from build123d import *

# Parameters (mm, degrees)
ESQUISSE1_R        = 1.6
BOSS_EXTRU_1_DEPTH = 1.6
CHANFREIN1_SIZE    = 0.2
CHANFREIN1_SIZE2   = 0.549495484
CHANFREIN2_SIZE    = 0.2
CHANFREIN2_SIZE2   = 0.549495484
ESQUISSE4_W        = 6.573690578
ESQUISSE4_H        = 5.811523554
BOSS_EXTRU_2_DEPTH = 2.5
ESQUISSE5_W        = 2.839601435
ESQUISSE5_H        = 2.289720849
ESQUISSE5_W_2      = 2.157836197
ESQUISSE5_H_2      = 2.945915503
ESQUISSE5_W_3      = 2.645694815
ESQUISSE5_H_3      = 1.363110326
ESQUISSE5_W_4      = 3.433774122
ESQUISSE5_H_4      = 3.640175845
ESQUISSE5_W_5      = 2.683222401
ESQUISSE5_H_5      = 0.956953443
BOSS_EXTRU_3_DEPTH = 2


with BuildPart() as part:
    # Esquisse1 → Boss.-Extru.1 (new body)
    with BuildSketch(Plane(origin=(0, 0, 0), x_dir=(1, 0, 0), z_dir=(0, 1, 0))):
        with BuildLine():
            Line((16.1, -18.1), (-16.1, -18.1))
            ThreePointArc((-16.1, -18.1), (-17.514213562, -17.514213562), (-18.1, -16.1))
            Line((-18.1, -16.1), (-18.1, 16.1))
            ThreePointArc((-18.1, 16.1), (-17.514213562, 17.514213562), (-16.1, 18.1))
            Line((-16.1, 18.1), (16.1, 18.1))
            ThreePointArc((16.1, 18.1), (17.514213562, 17.514213562), (18.1, 16.1))
            Line((18.1, 16.1), (18.1, -16.1))
            ThreePointArc((18.1, -16.1), (17.514213562, -17.514213562), (16.1, -18.1))
        make_face()
        with Locations((-15.25, 15.25)):
            Circle(ESQUISSE1_R, mode=Mode.SUBTRACT)
        with Locations((15.25, 15.25)):
            Circle(ESQUISSE1_R, mode=Mode.SUBTRACT)
        with Locations((15.25, -15.25)):
            Circle(ESQUISSE1_R, mode=Mode.SUBTRACT)
        with Locations((-15.25, -15.25)):
            Circle(ESQUISSE1_R, mode=Mode.SUBTRACT)
    extrude(amount=BOSS_EXTRU_1_DEPTH)

    # Chanfrein1
    chanfrein1_edges = [part.edges().sort_by_distance(p)[0] for p in [
        (17.514213562, 1.6, -17.514213562),
        (0, 1.6, -18.1),
        (-17.514213562, 1.6, -17.514213562),
        (-18.1, 1.6, 0),
        (-17.514213562, 1.6, 17.514213562),
        (0, 1.6, 18.1),
        (17.514213562, 1.6, 17.514213562),
        (18.1, 1.6, 0),
    ]]
    chanfrein1_side = [part.faces().sort_by_distance(p)[0] for p in [
        (0, 1.6, 0),
    ]]
    chamfer(chanfrein1_edges, length=CHANFREIN1_SIZE, length2=CHANFREIN1_SIZE2, reference=chanfrein1_side[0])

    # Chanfrein2
    chanfrein2_edges = [part.edges().sort_by_distance(p)[0] for p in [
        (18.1, 0, 0),
        (17.514213562, 0, 17.514213562),
        (0, 0, 18.1),
        (-17.514213562, 0, 17.514213562),
        (-18.1, 0, 0),
        (-17.514213562, 0, -17.514213562),
        (0, 0, -18.1),
        (17.514213562, 0, -17.514213562),
    ]]
    chanfrein2_side = [part.faces().sort_by_distance(p)[0] for p in [
        (0, 0, 0),
    ]]
    chamfer(chanfrein2_edges, length=CHANFREIN2_SIZE, length2=CHANFREIN2_SIZE2, reference=chanfrein2_side[0])

    # Esquisse4 → Boss.-Extru.2 (add)
    with BuildSketch(Plane(origin=(0, 1.6, 0), x_dir=(1, 0, 0), z_dir=(0, 1, 0))):
        with Locations((-6.049700749, -4.854717359)):
            Rectangle(ESQUISSE4_W, ESQUISSE4_H)
    extrude(amount=BOSS_EXTRU_2_DEPTH)

    # Esquisse5 → Boss.-Extru.3 (add)
    with BuildSketch(Plane(origin=(0, 1.6, 0), x_dir=(1, 0, 0), z_dir=(0, 1, 0))):
        with Locations((1.628867377, 4.102355057)):
            Rectangle(ESQUISSE5_W, ESQUISSE5_H)
        with Locations((5.922641632, 3.492800834)):
            Rectangle(ESQUISSE5_W_2, ESQUISSE5_H_2)
        with Locations((1.531914066, 0.681555163)):
            Rectangle(ESQUISSE5_W_3, ESQUISSE5_H_3)
        with Locations((1.49438648, -3.384129307)):
            Rectangle(ESQUISSE5_W_4, ESQUISSE5_H_4)
        with Locations((-7.080666928, 4.487281863)):
            Rectangle(ESQUISSE5_W_5, ESQUISSE5_H_5)
    extrude(amount=BOSS_EXTRU_3_DEPTH)


solid = part.part
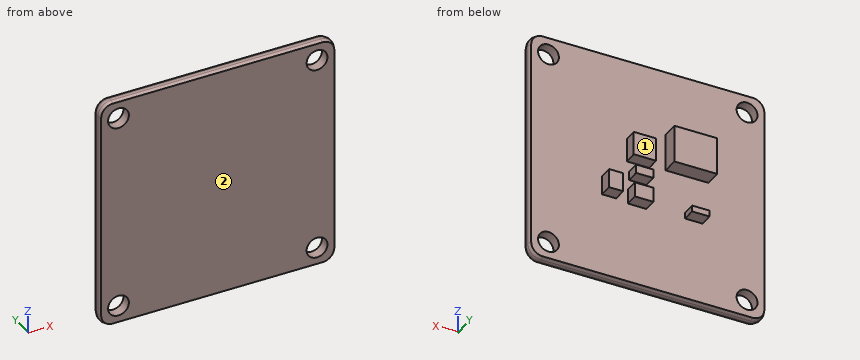
Build history of the part. All positions in model axes, mm. Face numbers are marked on the shaded views. A direction names the side the tool comes from. Round coordinates to 2 decimals unless told otherwise and drop trailing zeros. Loops run counter-clockwise (first coordinate to the right, second up) from the corner with the lowest first, then second, coordinate; pieces in that order, holes last. Notation, with made-up numbers: (72, -37) -> (92, -37) arc R15 ccw to (92, -12) -> close; hole circle Ø11 at (56, -27.75). An arc over 180 degrees is marked (long way). Answer in a Markdown table with one row per item.
Item 1: Which spindle directions (+Z, -Z, +X, -X, +Y, -Y) get a long thin tool onto all of the face, cutting with end or side? Do the marked faces 1 and 2. Say none if no direction does.
Answers below:
| item | result |
|---|---|
| face 1 | +Z, -Z, +X, +Y |
| face 2 | +Z, -Z, +X, -X, -Y |
Item 2: Drill centre lines: L1, parallel to X at y = 0.95, z = -15.25; L2, parallel to Z at x = 1.5, y = 3.2. Where is each one in solid material? Low to high. Write a range as [from, to].
Answers below:
| item | result |
|---|---|
| L1 | x = [-18.1, -16.85], [-13.65, 13.65], [16.85, 18.1] |
| L2 | z = [-5.25, -2.96], [-1.36, 0], [1.56, 5.2] |
Item 3: Saw through at C-C (z = 15.25). Write the cut outline in (x, y), and give its area (3 significant figures).
Answers below:
| item | result |
|---|---|
| outline | (-18.1, 0.55) -> (-17.9, 0) -> (-16.85, 0) -> (-16.85, 1.6) -> (-17.9, 1.6) -> (-18.1, 1.05) -> close; (-13.65, 0) -> (13.65, 0) -> (13.65, 1.6) -> (-13.65, 1.6) -> close; (16.85, 0) -> (17.9, 0) -> (18.1, 0.55) -> (18.1, 1.05) -> (17.9, 1.6) -> (16.85, 1.6) -> close |
| area | 47.5 mm² |
Item 4: Saw through at A-A (y = 3.1). Write the cut outline in (x, z).
Answers below:
| item | result |
|---|---|
| outline | (-9.34, 1.95) -> (-2.76, 1.95) -> (-2.76, 7.76) -> (-9.34, 7.76) -> close; (-8.42, -4.97) -> (-5.74, -4.97) -> (-5.74, -4.01) -> (-8.42, -4.01) -> close; (-0.22, 1.56) -> (3.21, 1.56) -> (3.21, 5.2) -> (-0.22, 5.2) -> close; (0.21, -5.25) -> (3.05, -5.25) -> (3.05, -2.96) -> (0.21, -2.96) -> close; (0.21, -1.36) -> (2.85, -1.36) -> (2.85, 0) -> (0.21, 0) -> close; (4.84, -4.97) -> (7, -4.97) -> (7, -2.02) -> (4.84, -2.02) -> close |
Item 5: Pin check, flat tips, straight feed: pin 1 (0.6 mm diameter, centred on y = 2, z = -4, fed in from -X); pin 2 (2 mm diameter, centred on y = 2.5, z = -8, fed in from -X); pin 3 (2 mm diameter, centred on x = -2, z = -2, fed in from -Y); pin 4 (1.6 mm diameter, centred on y = 2.5, z = 2.5, fed in from -X). Stop position of each tip, or through.
Answers below:
| item | result |
|---|---|
| pin 1 | stops at x = -8.42 |
| pin 2 | stops at x = -17.94 |
| pin 3 | stops at y = 0 |
| pin 4 | stops at x = -9.34 |
Item 6: Saw through at B-B (x = 15.25). Write the cut outline in (y, z).
Answers below:
| item | result |
|---|---|
| outline | (0, -17.9) -> (0.55, -18.1) -> (1.05, -18.1) -> (1.6, -17.9) -> (1.6, -16.85) -> (0, -16.85) -> close; (0, -13.65) -> (1.6, -13.65) -> (1.6, 13.65) -> (0, 13.65) -> close; (0, 16.85) -> (1.6, 16.85) -> (1.6, 17.9) -> (1.05, 18.1) -> (0.55, 18.1) -> (0, 17.9) -> close |
Item 7: Saw through at D-D (x = 6.5). Write the cut outline in (y, z), and give its area (3 significant figures).
Answers below:
| item | result |
|---|---|
| outline | (0, -17.9) -> (0.55, -18.1) -> (1.05, -18.1) -> (1.6, -17.9) -> (1.6, -4.97) -> (3.6, -4.97) -> (3.6, -2.02) -> (1.6, -2.02) -> (1.6, 17.9) -> (1.05, 18.1) -> (0.55, 18.1) -> (0, 17.9) -> close |
| area | 63.6 mm² |
